Read the model definition and answer for the solid it produces. Units are mm, in the model's axes. A direction names the side the tool comes from. Give positions to 0.01 mm unless a question says otherwise; leave off trailing zeros. Loops run counter-clockwise (first coordinate to the right, second up) from the corner with the lowest first, then second, coordinate; pieces in that order, holes last. Notation, with made-up numbers: (5, 34.5) - (48, 34.5) arc R36 ccw to (48, 72.5) - close; hole circle Ø9 at (15, 88.25). An arc over 180 degrees is marked (long way). Put each result on its own line as item: value. Start each with the question number.
1. For a pull along Z with two mould halves and no side action, classify faces 5 (the flat face through (0, -102.5, 0)), 6 (the flat face through (-7.31, -83.3, 0.1)), 7 (the conical face through (0.357, 16.239, 6.757)) as released by +Z, released by -Z, zero draft, split by the parting line, or undercut.
2. A cutting plane is placed at D-D, the plane y = -6. Determine the outline of the cut face in (x, z), plus the area to 3 significant figures.
3. Consider L1, parallel to X at y = -136.1, z = -5; L2, parallel to Z at x = 13.5, y = -127; L3, parallel to Y at x = -9.5, z = 5. Determine where each line is inside the solid, lowest interval first. Write a range as from..to.
4. For faces 1 (the flat face through (-11, -28, -7)), 2 (the flat face through (-11, -28, 7)), 3 (the flat face through (7.516, -83.76, 0.098)), 4 (the flat face through (-18.5, -121, 0)), determine the directions among +Z, -Z, +X, -X, +Y, -Y from which every point of the face is accessible in a straight line to the end or side of a thin tool.
5. Given pin 1 Ø5 at (x, z) = (24, -5) entering from -Y; pin 2 Ø8 at (x, z) = (-14.5, -4) entering from +Y; pin 3 Ø6 at (y, z) = (-69, 7.5) entering from -X; pin 4 Ø4 at (y, z) = (-88, 7) entering from -X, each flat-ended and moving along its own axis, determine where each tip first touches the part or whether it passes through.
6. A cutting plane is placed at C-C, the plane z = -5. Count the separate pieces of the cut face and the enclosed holes in it, plus the area to 3 significant figures.
7. A cutting plane is placed at A-A, the plane x = -24. Determine the outline of the cut face in (y, z).
8. A cutting plane is placed at B-B, the plane y = -92. Determine the outline of the cut face in (x, z), plus the area to 3 significant figures.
```python
from build123d import *

# Parameters (mm, degrees)
BOSS_EXTRUDE1_DEPTH = 7
SKETCH2_W           = 42
SKETCH2_H           = 25
BOSS_EXTRUDE2_DEPTH = 40
SHELL1_T            = -2.5
CUT_EXTRUDE5_REACH  = 144.903
SKETCH9_W           = 10
SKETCH9_H           = 25
BOSS_EXTRUDE3_DEPTH = 5
CUT_EXTRUDE6_REACH  = 151.018
SKETCH10_W          = 17
SKETCH10_H          = 10
CUT_EXTRUDE8_REACH  = 146.196
CUT_EXTRUDE9_REACH  = 165.98
SKETCH13_R          = 2.1
CHAMFER1_SIZE       = 5


with BuildPart() as part:
    # Sketch1 → Boss-Extrude1 (new, symmetric)
    with BuildSketch(Plane.XY):
        with BuildLine():
            Line((-21, 0), (-21, -100))
            Line((-21, -100), (21, -100))
            Line((21, -100), (21, 0))
            ThreePointArc((21, 0), (0, 21), (-21, 0))
        make_face()
    extrude(amount=BOSS_EXTRUDE1_DEPTH, both=True)


with BuildPart() as body_2:
    # Sketch2 → Boss-Extrude2 (new body)
    with BuildSketch(Plane.XZ.offset(100)):
        Rectangle(SKETCH2_W, SKETCH2_H)
    extrude(amount=BOSS_EXTRUDE2_DEPTH)

    # Shell1
    shell1_openings = [body_2.faces().sort_by_distance(p)[0] for p in [
        (0, -140, 0),
    ]]
    offset(amount=SHELL1_T, openings=shell1_openings, kind=Kind.INTERSECTION)


with BuildPart() as part_1:
    add(part.part)

    # Combine1: union body 2
    add(body_2.part)

    # Sketch8 → Cut-Extrude5 (cut, up to next)
    with BuildSketch(Plane.XY.offset(7), mode=Mode.PRIVATE) as cut_extrude5_sk1:
        with BuildLine():
            ThreePointArc((-3.75, 0), (-5, 1.25), (-6.25, 0))
            Line((-6.25, 0), (-3.75, 0))
        make_face()
    cut_extrude5_tool1 = extrude(cut_extrude5_sk1.sketch, amount=-CUT_EXTRUDE5_REACH, mode=Mode.PRIVATE) & part_1.part
    # Sketch8 → Cut-Extrude5 (cut, up to next)
    with BuildSketch(Plane.XY.offset(7), mode=Mode.PRIVATE) as cut_extrude5_sk2:
        with BuildLine():
            Line((-3.75, 0), (-6.25, 0))
            ThreePointArc((-6.25, 0), (-5, -1.25), (-3.75, 0))
        make_face()
    cut_extrude5_tool2 = extrude(cut_extrude5_sk2.sketch, amount=-CUT_EXTRUDE5_REACH, mode=Mode.PRIVATE) & part_1.part
    # Sketch8 → Cut-Extrude5 (cut, up to next)
    with BuildSketch(Plane.XY.offset(7), mode=Mode.PRIVATE) as cut_extrude5_sk3:
        with BuildLine():
            ThreePointArc((-3.75, 0), (-5, 1.25), (-6.25, 0))
            Line((-6.25, 0), (-3.75, 0))
        make_face()
    cut_extrude5_tool3 = extrude(cut_extrude5_sk3.sketch, amount=-CUT_EXTRUDE5_REACH, mode=Mode.PRIVATE) & part_1.part
    # Sketch8 → Cut-Extrude5 (cut, up to next)
    with BuildSketch(Plane.XY.offset(7), mode=Mode.PRIVATE) as cut_extrude5_sk4:
        with BuildLine():
            Line((-3.75, 0), (-6.25, 0))
            ThreePointArc((-6.25, 0), (-5, -1.25), (-3.75, 0))
        make_face()
    cut_extrude5_tool4 = extrude(cut_extrude5_sk4.sketch, amount=-CUT_EXTRUDE5_REACH, mode=Mode.PRIVATE) & part_1.part
    # Sketch8 → Cut-Extrude5 (cut, up to next)
    with BuildSketch(Plane.XY.offset(7), mode=Mode.PRIVATE) as cut_extrude5_sk5:
        with BuildLine():
            ThreePointArc((3.75, 0), (5, -1.25), (6.25, 0))
            Line((6.25, 0), (3.75, 0))
        make_face()
    cut_extrude5_tool5 = extrude(cut_extrude5_sk5.sketch, amount=-CUT_EXTRUDE5_REACH, mode=Mode.PRIVATE) & part_1.part
    # Sketch8 → Cut-Extrude5 (cut, up to next)
    with BuildSketch(Plane.XY.offset(7), mode=Mode.PRIVATE) as cut_extrude5_sk6:
        with BuildLine():
            Line((3.75, 0), (6.25, 0))
            ThreePointArc((6.25, 0), (5, 1.25), (3.75, 0))
        make_face()
    cut_extrude5_tool6 = extrude(cut_extrude5_sk6.sketch, amount=-CUT_EXTRUDE5_REACH, mode=Mode.PRIVATE) & part_1.part
    # Sketch8 → Cut-Extrude5 (cut, up to next)
    with BuildSketch(Plane.XY.offset(7), mode=Mode.PRIVATE) as cut_extrude5_sk7:
        with BuildLine():
            ThreePointArc((3.75, 0), (5, -1.25), (6.25, 0))
            Line((6.25, 0), (3.75, 0))
        make_face()
    cut_extrude5_tool7 = extrude(cut_extrude5_sk7.sketch, amount=-CUT_EXTRUDE5_REACH, mode=Mode.PRIVATE) & part_1.part
    # Sketch8 → Cut-Extrude5 (cut, up to next)
    with BuildSketch(Plane.XY.offset(7), mode=Mode.PRIVATE) as cut_extrude5_sk8:
        with BuildLine():
            Line((3.75, 0), (6.25, 0))
            ThreePointArc((6.25, 0), (5, 1.25), (3.75, 0))
        make_face()
    cut_extrude5_tool8 = extrude(cut_extrude5_sk8.sketch, amount=-CUT_EXTRUDE5_REACH, mode=Mode.PRIVATE) & part_1.part
    # Sketch8 → Cut-Extrude5 (cut, up to next)
    with BuildSketch(Plane.XY.offset(7), mode=Mode.PRIVATE) as cut_extrude5_sk9:
        with BuildLine():
            ThreePointArc((-2.5, 0), (0, -2.5), (2.5, 0))
            Line((2.5, 0), (-2.5, 0))
        make_face()
    cut_extrude5_tool9 = extrude(cut_extrude5_sk9.sketch, amount=-CUT_EXTRUDE5_REACH, mode=Mode.PRIVATE) & part_1.part
    # Sketch8 → Cut-Extrude5 (cut, up to next)
    with BuildSketch(Plane.XY.offset(7), mode=Mode.PRIVATE) as cut_extrude5_sk10:
        with BuildLine():
            Line((-2.5, 0), (2.5, 0))
            ThreePointArc((2.5, 0), (0, 2.5), (-2.5, 0))
        make_face()
    cut_extrude5_tool10 = extrude(cut_extrude5_sk10.sketch, amount=-CUT_EXTRUDE5_REACH, mode=Mode.PRIVATE) & part_1.part
    # Sketch8 → Cut-Extrude5 (cut, up to next)
    with BuildSketch(Plane.XY.offset(7), mode=Mode.PRIVATE) as cut_extrude5_sk11:
        with BuildLine():
            ThreePointArc((-2.5, 0), (0, -2.5), (2.5, 0))
            Line((2.5, 0), (-2.5, 0))
        make_face()
    cut_extrude5_tool11 = extrude(cut_extrude5_sk11.sketch, amount=-CUT_EXTRUDE5_REACH, mode=Mode.PRIVATE) & part_1.part
    # Sketch8 → Cut-Extrude5 (cut, up to next)
    with BuildSketch(Plane.XY.offset(7), mode=Mode.PRIVATE) as cut_extrude5_sk12:
        with BuildLine():
            Line((-2.5, 0), (2.5, 0))
            ThreePointArc((2.5, 0), (0, 2.5), (-2.5, 0))
        make_face()
    cut_extrude5_tool12 = extrude(cut_extrude5_sk12.sketch, amount=-CUT_EXTRUDE5_REACH, mode=Mode.PRIVATE) & part_1.part
    add(cut_extrude5_tool1.solids().sort_by_distance((-5, 0.530516, 7))[0], mode=Mode.SUBTRACT)
    add(cut_extrude5_tool2.solids().sort_by_distance((-5, -0.530516, 7))[0], mode=Mode.SUBTRACT)
    add(cut_extrude5_tool3.solids().sort_by_distance((-5, 0.530516, 7))[0], mode=Mode.SUBTRACT)
    add(cut_extrude5_tool4.solids().sort_by_distance((-5, -0.530516, 7))[0], mode=Mode.SUBTRACT)
    add(cut_extrude5_tool5.solids().sort_by_distance((5, -0.530516, 7))[0], mode=Mode.SUBTRACT)
    add(cut_extrude5_tool6.solids().sort_by_distance((5, 0.530516, 7))[0], mode=Mode.SUBTRACT)
    add(cut_extrude5_tool7.solids().sort_by_distance((5, -0.530516, 7))[0], mode=Mode.SUBTRACT)
    add(cut_extrude5_tool8.solids().sort_by_distance((5, 0.530516, 7))[0], mode=Mode.SUBTRACT)
    add(cut_extrude5_tool9.solids().sort_by_distance((0, -1.061033, 7))[0], mode=Mode.SUBTRACT)
    add(cut_extrude5_tool10.solids().sort_by_distance((0, 1.061033, 7))[0], mode=Mode.SUBTRACT)
    add(cut_extrude5_tool11.solids().sort_by_distance((0, -1.061033, 7))[0], mode=Mode.SUBTRACT)
    add(cut_extrude5_tool12.solids().sort_by_distance((0, 1.061033, 7))[0], mode=Mode.SUBTRACT)

    # Sketch9 → Boss-Extrude3 (add)
    with BuildSketch(Plane.XZ.offset(140)):
        with Locations((-23.5, 0)):
            Rectangle(SKETCH9_W, SKETCH9_H)
        with Locations((23.5, 0)):
            Rectangle(SKETCH9_W, SKETCH9_H)
    extrude(amount=-BOSS_EXTRUDE3_DEPTH)

    # Sketch10 → Cut-Extrude6 (cut, up to next)
    with BuildSketch(Plane(origin=(21, 0, 0), x_dir=(0, 0, -1), z_dir=(1, 0, 0)), mode=Mode.PRIVATE) as cut_extrude6_sk1:
        with Locations((0, -115)):
            Rectangle(SKETCH10_W, SKETCH10_H)
    cut_extrude6_tool1 = extrude(cut_extrude6_sk1.sketch, amount=-CUT_EXTRUDE6_REACH, mode=Mode.PRIVATE) & part_1.part
    add(cut_extrude6_tool1.solids().sort_by_distance((21, -115, 0))[0], mode=Mode.SUBTRACT)

    # Sketch12 → Cut-Extrude8 (cut, up to next)
    with BuildSketch(Plane.XY.offset(7), mode=Mode.PRIVATE) as cut_extrude8_sk1:
        Polygon((14.82390073, -17.057998377), (0, -50), (-14.82390073, -17.057998377), align=None)
    cut_extrude8_tool1 = extrude(cut_extrude8_sk1.sketch, amount=-CUT_EXTRUDE8_REACH, mode=Mode.PRIVATE) & part_1.part
    # Sketch12 → Cut-Extrude8 (cut, up to next)
    with BuildSketch(Plane.XY.offset(7), mode=Mode.PRIVATE) as cut_extrude8_sk2:
        Polygon((-14.82390073, -34.115996755), (-3.838049635, -58.528999189), (-14.82390073, -82.942001623), align=None)
    cut_extrude8_tool2 = extrude(cut_extrude8_sk2.sketch, amount=-CUT_EXTRUDE8_REACH, mode=Mode.PRIVATE) & part_1.part
    # Sketch12 → Cut-Extrude8 (cut, up to next)
    with BuildSketch(Plane.XY.offset(7), mode=Mode.PRIVATE) as cut_extrude8_sk3:
        Polygon((14.82390073, -100), (0, -67.057998377), (-14.82390073, -100), align=None)
    cut_extrude8_tool3 = extrude(cut_extrude8_sk3.sketch, amount=-CUT_EXTRUDE8_REACH, mode=Mode.PRIVATE) & part_1.part
    # Sketch12 → Cut-Extrude8 (cut, up to next)
    with BuildSketch(Plane.XY.offset(7), mode=Mode.PRIVATE) as cut_extrude8_sk4:
        Polygon((14.82390073, -34.115996755), (14.82390073, -82.942001623), (3.838049635, -58.528999189), align=None)
    cut_extrude8_tool4 = extrude(cut_extrude8_sk4.sketch, amount=-CUT_EXTRUDE8_REACH, mode=Mode.PRIVATE) & part_1.part
    add(cut_extrude8_tool1.solids().sort_by_distance((0, -28.038666, 7))[0], mode=Mode.SUBTRACT)
    add(cut_extrude8_tool2.solids().sort_by_distance((-11.16195, -58.528999, 7))[0], mode=Mode.SUBTRACT)
    add(cut_extrude8_tool3.solids().sort_by_distance((0, -89.019333, 7))[0], mode=Mode.SUBTRACT)
    add(cut_extrude8_tool4.solids().sort_by_distance((11.16195, -58.528999, 7))[0], mode=Mode.SUBTRACT)

    # Sketch13 → Cut-Extrude9 (cut, up to next)
    with BuildSketch(Plane.XZ.offset(140), mode=Mode.PRIVATE) as cut_extrude9_sk1:
        with Locations(Location((-24, 5, 0), (0, 0, 270))):
            Circle(SKETCH13_R)
    cut_extrude9_tool1 = extrude(cut_extrude9_sk1.sketch, amount=-CUT_EXTRUDE9_REACH, mode=Mode.PRIVATE) & part_1.part
    # Sketch13 → Cut-Extrude9 (cut, up to next)
    with BuildSketch(Plane.XZ.offset(140), mode=Mode.PRIVATE) as cut_extrude9_sk2:
        with Locations(Location((-24, -5, 0), (0, 0, 270))):
            Circle(SKETCH13_R)
    cut_extrude9_tool2 = extrude(cut_extrude9_sk2.sketch, amount=-CUT_EXTRUDE9_REACH, mode=Mode.PRIVATE) & part_1.part
    # Sketch13 → Cut-Extrude9 (cut, up to next)
    with BuildSketch(Plane.XZ.offset(140), mode=Mode.PRIVATE) as cut_extrude9_sk3:
        with Locations(Location((24, 5, 0), (0, 0, 270))):
            Circle(SKETCH13_R)
    cut_extrude9_tool3 = extrude(cut_extrude9_sk3.sketch, amount=-CUT_EXTRUDE9_REACH, mode=Mode.PRIVATE) & part_1.part
    # Sketch13 → Cut-Extrude9 (cut, up to next)
    with BuildSketch(Plane.XZ.offset(140), mode=Mode.PRIVATE) as cut_extrude9_sk4:
        with Locations(Location((24, -5, 0), (0, 0, 270))):
            Circle(SKETCH13_R)
    cut_extrude9_tool4 = extrude(cut_extrude9_sk4.sketch, amount=-CUT_EXTRUDE9_REACH, mode=Mode.PRIVATE) & part_1.part
    add(cut_extrude9_tool1.solids().sort_by_distance((-24, -140, 5))[0], mode=Mode.SUBTRACT)
    add(cut_extrude9_tool2.solids().sort_by_distance((-24, -140, -5))[0], mode=Mode.SUBTRACT)
    add(cut_extrude9_tool3.solids().sort_by_distance((24, -140, 5))[0], mode=Mode.SUBTRACT)
    add(cut_extrude9_tool4.solids().sort_by_distance((24, -140, -5))[0], mode=Mode.SUBTRACT)

    # Chamfer1
    chamfer1_edges = [part_1.edges().sort_by_distance(p)[0] for p in [
        (21, -50, 7),
        (0, 21, 7),
        (21, -50, -7),
        (-21, -50, -7),
        (0, 21, -7),
        (-21, -50, 7),
    ]]
    chamfer(chamfer1_edges, length=CHAMFER1_SIZE)


solid = part_1.part
```
Return value:
1. face 5: undercut
1. face 6: zero draft
1. face 7: released by +Z
2. outline: (-21, -2) - (-16, -7) - (16, -7) - (21, -2) - (21, 2) - (16, 7) - (-16, 7) - (-21, 2) - close
2. area: 538 mm2
3. L1: x = -28.5..-26.1, -21.9..-18.5, 18.5..21.9, 26.1..28.5
3. L2: z = -12.5..-10, 10..12.5
3. L3: y = -102.5..-100, -88.17..-71.11, -45.95..-28.89, -17.06..15.29
4. face 1: -Z, +X, -X, +Y
4. face 2: +Z, +X, -X, +Y
4. face 3: +Z, -Z
4. face 4: -Y
5. pin 1: stops at y = -140
5. pin 2: stops at y = 17.87
5. pin 3: stops at x = -18.5
5. pin 4: stops at x = -18
6. separate pieces: 4
6. enclosed holes: 7
6. area: 2,870 mm2
7. outline: (-140, -12.5) - (-135, -12.5) - (-135, -7.1) - (-140, -7.1) - close; (-140, -2.9) - (-135, -2.9) - (-135, 2.9) - (-140, 2.9) - close; (-140, 7.1) - (-135, 7.1) - (-135, 12.5) - (-140, 12.5) - close
8. outline: (-21, -2) - (-16, -7) - (-11.22, -7) - (-11.22, 7) - (-16, 7) - (-21, 2) - close; (11.22, -7) - (16, -7) - (21, -2) - (21, 2) - (16, 7) - (11.22, 7) - close
8. area: 224 mm2
